For this review, take the finished solid that the model builds, in its own axes (mm). Face numbers are marked on the shaded views. A direction names the side the tool comes from. Give positions to 0.01 mm unless a question says otherwise; leave off trailing zeros. Write each loop counter-clockwise with the first axis right and the second up, starting at its lowest first coordinate (ties: lowest second). Pieces come first, ordered by that corner, then holes. Notation, with made-up numbers: M 5,18 L 39,18 A15 cw 39,42 Z; hole C -29,80 d3. An arc over 180 degrees is marked long. Use one line per item in the form item = value. Start each with the question number.
Q1. Consider section D-D on z = -4.5. Write out the cut boundary in (x, y) (3 decimals).
Q2. Consider section A-A on y = 0. Write out the cut boundary in (x, z) (3 decimals), and give its area (3 significant figures).
Q3. For probe 1 along X at (y, z) = (1.25, -6.25) (3 decimals); probe 2 along X at (y, z) = (0.25, 2.25); probe 3 along Y at (x, z) = (-12, -3), list the stretches that pass through material, from the lowest coordinate up. Write a range as [from, to].
Q4. Tool access review of the marked faces 1 and 2: name each direction out of +Z, -Z, +X, -X, +Y, -Y from which nothing blocks a thin tool from reaching the whole face with its end or side.
Q5. Consider section C-C on x = -88. Write out the cut boundary in (y, z).
Q6. Clearance check with flat-ended pins moving along their axes: pin 1 Ø1 at (x, y) = (-17.5, 1.5) entering from -Z; pin 2 Ø8 at (x, y) = (-14, -1.5) entering from -Z; pin 3 Ø1 at (x, y) = (-12.5, -3) entering from +Z; pin 4 Ø8 at (x, y) = (-91.5, 0) entering from -Z. State where each tip first meets the part, or that it passes through.
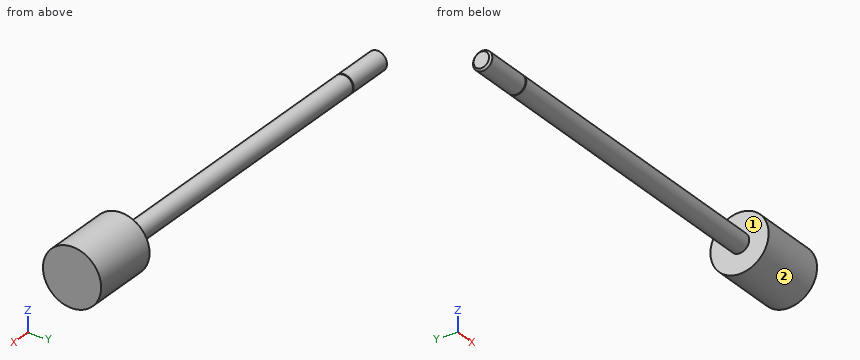
Autodesk Inventor part; units mm, degrees
ref_plane "h1_XY" through (-108.7374, 0, 0) normal (0, 1, 0) x (1, 0, 0)
ref_plane "h1_YZ" through (-108.7374, 0, 0) normal (1, 0, 0) x (0, 0, -1)
ref_plane "h1_ZX" through (-108.7374, 0, 0) normal (0, 0, -1) x (0, 1, 0)
sketch "Sketch_3" plane through (0, 0, 0) normal (0, 0, 1) x (1, 0, 0)
  line L0 (0, 0) -> (-108.7374, 0)
  line L1 (-108.7374, 0) -> (-108.7374, 1.9406)
  line L2 (-108.7374, 1.9406) -> (-108.265, 2.413)
  line L3 (-108.265, 2.413) -> (0, 2.413)
  line L4 (0, 2.413) -> (0, 0)
  line L5 (0, 0) -> (-108.7374, 0)
revolve "Revolution1" add sketch "Sketch_3" angle 360 about axis through (0, 0, 0) along (1, 0, 0)
thread "Thread1"
sketch "Sketch_17" plane through (0, 0, 0) normal (0, 0, 1) x (1, 0, 0)
  line L0 (108.7374, 0) -> (-108.7374, 0)
  line L1 (-96.2914, 2.413) -> (-96.2914, 2.159)
  line L2 (-96.2914, 2.159) -> (-96.0374, 2.159)
  line L3 (-96.0374, 2.159) -> (-96.0374, 2.413)
  line L4 (-96.0374, 2.413) -> (-96.2914, 2.413)
revolve "Revolution2" cut sketch "Sketch_17" angle 360 about axis through (108.7374, 0, 0) along (1, 0, 0)
sketch "Sketch_12" plane through (0, 0, 0) normal (0, 0, 1) x (1, 0, 0)
  line L0 (1.524, 0) -> (-15.875, 0)
  line L1 (-15.875, 0) -> (-15.875, 7.2771)
  line L2 (-15.875, 7.2771) -> (1.524, 7.2771)
  line L3 (1.524, 7.2771) -> (1.524, 0)
  line L4 (1.524, 0) -> (-15.875, 0)
revolve "Revolution3" add sketch "Sketch_12" angle 360 about axis through (1.524, 0, 0) along (1, 0, 0)
ref_plane "h1_XY" through (-108.7374, 0, 0) normal (0, 1, 0) x (1, 0, 0)
ref_plane "h1_YZ" through (-108.7374, 0, 0) normal (1, 0, 0) x (0, 0, -1)
ref_plane "h1_ZX" through (-108.7374, 0, 0) normal (0, 0, -1) x (0, 1, 0)
ref_plane "h2_XY" through (-96.0374, 0, 0) normal (0, 1, 0) x (1, 0, 0)
ref_plane "h2_YZ" through (-96.0374, 0, 0) normal (1, 0, 0) x (0, 0, -1)
ref_plane "h2_ZX" through (-96.0374, 0, 0) normal (0, 0, -1) x (0, 1, 0)
ref_plane "k1_XY" through (-108.7374, 0, -2.413) normal (0, 1, 0) x (1, 0, 0)
ref_plane "k1_YZ" through (-108.7374, 0, -2.413) normal (1, 0, 0) x (0, 0, -1)
ref_plane "k1_ZX" through (-108.7374, 0, -2.413) normal (0, 0, -1) x (0, 1, 0)
ref_plane "k2_XY" through (-108.7374, 0, 2.413) normal (0, 1, 0) x (1, 0, 0)
ref_plane "k2_YZ" through (-108.7374, 0, 2.413) normal (1, 0, 0) x (0, 0, -1)
ref_plane "k2_ZX" through (-108.7374, 0, 2.413) normal (0, 0, -1) x (0, 1, 0)
ref_plane "start_XY" through (-96.0374, 0, 0) normal (0, 1, 0) x (1, 0, 0)
ref_plane "start_YZ" through (-96.0374, 0, 0) normal (1, 0, 0) x (0, 0, -1)
ref_plane "start_ZX" through (-96.0374, 0, 0) normal (0, 0, -1) x (0, 1, 0)
ref_plane "to_prc_XY" through (-96.0374, 0, 0) normal (1, 0, 0) x (0, 0, -1)
ref_plane "to_prc_YZ" through (-96.0374, 0, 0) normal (0, 0, -1) x (0, 1, 0)
ref_plane "to_prc_ZX" through (-96.0374, 0, 0) normal (0, 1, 0) x (1, 0, 0)
ref_plane "to_rod_guide_XY" through (-108.7374, 0, 0) normal (1, 0, 0) x (0, 0, -1)
ref_plane "to_rod_guide_YZ" through (-108.7374, 0, 0) normal (0, 0, -1) x (0, 1, 0)
ref_plane "to_rod_guide_ZX" through (-108.7374, 0, 0) normal (0, 1, 0) x (1, 0, 0)
properties part number "D-75080.5-1.5XP-4.281-3pos"
Working result:
q1.outline = M -15.875,-5.719 L 1.524,-5.719 L 1.524,5.719 L -15.875,5.719 Z
q2.outline = M -108.737,-1.941 L -108.265,-2.413 L -96.291,-2.413 L -96.291,-2.159 L -96.037,-2.159 L -96.037,-2.413 L -15.875,-2.413 L -15.875,-7.277 L 1.524,-7.277 L 1.524,7.277 L -15.875,7.277 L -15.875,2.413 L -96.037,2.413 L -96.037,2.159 L -96.291,2.159 L -96.291,2.413 L -108.265,2.413 L -108.737,1.941 Z
q2.area = 701 mm²
q3.probe_1 = [-15.875, 1.524]
q3.probe_2 = [-108.41, -96.29], [-96.04, 1.52]
q3.probe_3 = [-6.63, 6.63]
q4.face_1 = -X
q4.face_2 = +X, -X
q5.outline = C 0,0 d4.83
q6.pin_1 = -2.2
q6.pin_2 = -7.28
q6.pin_3 = 6.83
q6.pin_4 = -2.41
